The model under review builds one solid part; all positions refer to its coordinate system, in mm. A direction names the side the tool comes from. Round coordinates to 2 decimals unless told otherwise and drop trailing zeros. Write each loop counter-clockwise with the first axis right and the second up, starting at its lowest first coordinate (ties: lowest second). Pieces come first, ordered by that corner, then holes. Notation, with made-up numbers: (19, -14.5) -> (78, -14.5) arc R38 cw to (78, 24.5) -> close; hole circle Ø1 at (84, -15.5). An arc over 180 degrees is marked (long way). Return JSON: item names as keys, results as strings. Group by question number.
1. Take a section at B-B, the plane z = 0. Write out the cut boundary in (x, y), then the cut area to 3 significant figures.
2. Mouldability with a two-part tool opening along X and no side actions: class faces 1 (the cylindrical face through (-2.17, -75.07, -9.76)), 2 (the flat face through (-30, 3, 28)), 3 (the flat face through (0, -70, 13)) as pulls with the +X half, pulls with the -X half, needs draft (parallel to the pull), parting line crosses it, or undercut.
3. For line 1 along Z through (x, y) = (0, -76.75); line 2 along Y through (x, z) = (-15.5, -5); line 3 along Z through (x, y) = (15, -60.5), list the stretches that pass through material, from the lowest coordinate up. Write a range as from..to.
4. Tool access review of faces 4 (the flat face through (0, 5, 0)), 5 (the flat face through (0, 0, 12)), 6 (the flat face through (0, -80, 18)): name each direction out of +Z, -Z, +X, -X, +Y, -Y from which nothing blocks a thin tool from reaching the whole face with its end or side.
5. Take a section at A-A, the plane x = 0. Write out the cut boundary in (y, z), then the cut area to 3 significant figures.
6. Clearance check with flat-ended pins moving along their axes: P1, Ø5, axis at x = -17.5, y = -44.5, coming from the -Z side; P2, Ø18, axis at x = 0, z = 0, coming from the -Y side; P3, Ø5, axis at y = -4.5, z = 16.5, coming from the +X side. State where each tip first meets the part, or that it passes through.
7. Take a section at D-D, the plane y = 8. Write out the cut boundary in (x, z), then the cut area to 3 significant figures.
8. Take a section at C-C, the plane z = 44.5. Write out the cut boundary in (x, y).
Autodesk Fusion 360 part; units mm, degrees
sketch "草图1" plane through (0, 0, 0) normal (0, 1, 0) x (1, 0, 0) in component "Component"
  line L0 (-30, 25) -> (30, 25)
  line L1 (30, 25) -> (30, -60)
  line L2 (30, -60) -> (-30, -60)
  line L3 (-30, -60) -> (-30, 25)
  dimension "d1" = 60
  dimension "d2" = 85
  dimension "d3" = 25
  dimension "d4" = 30
extrude "拉伸1" add sketch "草图1" along normal blind 10 in component "Component"
sketch "草图2" plane through (0, 0, 0) normal (0, -1, 0) x (1, 0, 0) in component "Component"
  line L0 (30, 60) -> (-30, 60)
  line L1 (-30, 60) -> (-30, -25)
  line L2 (-30, -25) -> (30, -25)
  line L3 (30, -25) -> (30, 60)
  line L4 (-30, 60) -> (30, 60)
  line L5 (30, 60) -> (30, 50)
  line L6 (30, 50) -> (-30, 50)
  line L7 (-30, 50) -> (-30, 60)
  dimension "d8" = 10
extrude "拉伸2" add sketch "草图2" along normal blind 80 contours L0 L1 L3 L4 L5 L6 L7 in component "Component"
sketch "草图3" plane through (0, 0, 50) normal (0, 0, -1) x (-1, 0, 0) in component "Component"
  line L0 (30, 0) -> (-30, 0)
  line L1 (-30, 0) -> (-30, -80)
  line L2 (-30, -80) -> (30, -80)
  line L3 (30, -80) -> (30, 0)
  line L4 (-30, -70) -> (30, -70)
  line L5 (30, -70) -> (30, -80)
  line L6 (30, -80) -> (-30, -80)
  line L7 (-30, -80) -> (-30, -70)
  dimension "d11" = 10
extrude "拉伸3" add sketch "草图3" along normal blind 75 contours L1 L2 L3 L4 L5 L6 L7 in component "Component"
sketch "草图4" plane through (0, -80, 0) normal (0, -1, 0) x (1, 0, 0) in component "Component"
  line L0 (30, -25) -> (30, 60)
  line L1 (30, 60) -> (-30, 60)
  line L2 (-30, 60) -> (-30, -25)
  line L3 (-30, -25) -> (30, -25)
  circle A0 centre (0, 0) radius 10
  dimension "d14" = 20
extrude "拉伸4" cut sketch "草图4" against normal blind 10 contours A0 in component "Component"
thread "螺纹1" in component "Component"
extrude "拉伸5" add 1 faces at (-10, 10, 3.3333) along direction (0, 1, 0) blind 10 in component "Component"
sketch "草图5" plane through (0, 20, 0) normal (0, 1, 0) x (-1, 0, 0) in component "Component"
  line L0 (30, 60) -> (-30, 60)
  line L1 (-30, 60) -> (-30, -25)
  line L2 (-30, -25) -> (30, -25)
  line L3 (30, -25) -> (30, 60)
  circle A0 centre (0, 0) radius 10
extrude "拉伸6" cut sketch "草图5" against normal blind 15 contours A0 in component "Component"
component "Component" placed x (1, 0, 0) y (0, 1, 0) z (0, 0, 1) at (0, 0, 0)
Output:
{
 "1": {"outline": "(-30, -80) -> (-10, -80) -> (-10, -70) -> (-30, -70) -> close; (-30, 0) -> (30, 0) -> (30, 20) -> (10, 20) -> (10, 5) -> (-10, 5) -> (-10, 20) -> (-30, 20) -> close; (10, -80) -> (30, -80) -> (30, -70) -> (10, -70) -> close", "area": "1,300 mm^2"},
 "2": {"face 1": "undercut", "face 2": "pulls with the -X half", "face 3": "needs draft"},
 "3": {"line 1": "z = -25..-10, 10..60", "line 2": "y = -80..-70, 0..20", "line 3": "z = 50..60"},
 "4": {"face 4": "+Y", "face 5": "-Z, +X, -X", "face 6": "+Z, -Z, +X, -X, -Y"},
 "5": {"outline": "(-80, -25) -> (-70, -25) -> (-70, -10) -> (-80, -10) -> close; (-80, 10) -> (-70, 10) -> (-70, 50) -> (0, 50) -> (0, -25) -> (20, -25) -> (20, -10) -> (5, -10) -> (5, 10) -> (20, 10) -> (20, 60) -> (-80, 60) -> close", "area": "2,750 mm^2"},
 "6": {"P1": "stops at z = 50", "P2": "stops at y = 0", "P3": "passes through"},
 "7": {"outline": "(-30, -25) -> (30, -25) -> (30, 60) -> (-30, 60) -> close; hole circle Ø20 at (0, 0)", "area": "4,790 mm^2"},
 "8": {"outline": "(-30, -80) -> (30, -80) -> (30, -70) -> (-30, -70) -> close; (-30, 0) -> (30, 0) -> (30, 20) -> (-30, 20) -> close"}
}
